from build123d import *

# Parameters (mm, degrees)
REVOLUTION_ANGLE = 100
FILLET_R         = 8
PAD_DEPTH        = 8
POCKET_DEPTH     = 2
CHAMFER_SIZE     = 1
SKETCH005_W      = 3
SKETCH005_H      = 7
POCKET001_DEPTH  = 81.861582
POCKET002_DEPTH  = 78.501
FILLET001_R      = 3
FILLET002_R      = 1


with BuildPart() as part:
    # Sketch → Revolution (revolve, symmetric)
    with BuildSketch(Plane.XY) as revolution_sk:
        with BuildLine():
            ThreePointArc((28, 223.488706), (0, 250), (-28, 223.488706))
            Line((-34.75, 100), (-28, 223.488706))
            Line((-34.75, 100), (-32.5, 100))
            Line((-32.5, 100), (-25.552843, 224))
            ThreePointArc((25.552843, 224), (0, 248.161305), (-25.552843, 224))
            Line((25.552843, 224), (32.5, 100))
            Line((32.5, 100), (34.75, 100))
            Line((34.75, 100), (28, 223.488706))
        make_face()
    revolve(axis=Axis((0, 0, 0), (1, 0, 0)), revolution_arc=REVOLUTION_ANGLE / 2)
    revolve(revolution_sk.sketch, axis=Axis((0, 0, 0), (-1, 0, 0)), revolution_arc=REVOLUTION_ANGLE / 2)

    # Fillet
    fillet_edges = [part.edges().sort_by_distance(p)[0] for p in [
        (33.625, 64.278761, 76.604444),
        (-33.625, 64.278761, 76.604444),
    ]]
    fillet(fillet_edges, radius=FILLET_R)

    # Sketch002 (on Face5 of Fillet) → Pad (new body)
    with BuildSketch(Plane(origin=(0, 0, 0), x_dir=(1, 0, 0), z_dir=(0, -0.766044, 0.642788))):
        Polygon((-43.394171, 132.697505), (-46.5, 121.106395), (-33.248819, 107.855214), (-31, 145.091677), align=None)
        Polygon((43.394171, 132.697505), (46.5, 121.106395), (33.248819, 107.855214), (31, 145.091677), align=None)
        Polygon((28, 194.106395), (32, 198.106395), (32, 206.106395), (28, 210.106395), (24, 206.106395), (24, 198.106395), align=None)
        Polygon((-28, 194.106395), (-24, 198.106395), (-24, 206.106395), (-28, 210.106395), (-32, 206.106395), (-32, 198.106395), align=None)
    extrude(amount=-PAD_DEPTH)

    # Sketch003 (on Face47 of Pad) → Pocket (cut)
    with BuildSketch(Plane(origin=(0, 0, 0), x_dir=(1, 0, 0), z_dir=(0, -0.766044, 0.642788))):
        Polygon((35, 146.869795), (45, 97.88), (47.939388, 98.48), (37.939388, 147.469795), align=None)
        Polygon((-47.939388, 98.48), (-45, 97.88), (-35, 146.869795), (-37.939388, 147.469795), align=None)
    extrude(amount=-POCKET_DEPTH, mode=Mode.SUBTRACT)

    # Chamfer
    chamfer_edges = [part.edges().sort_by_distance(p)[0] for p in [
        (42.094426, 81.707526, 97.375238),
        (38.89944, 82.126736, 97.874832),
        (-38.89944, 82.126736, 97.874832),
        (-42.094426, 81.707526, 97.375238),
    ]]
    chamfer(chamfer_edges, length=CHAMFER_SIZE)

    # Sketch005 (on Face6 of Chamfer) → Pocket001 (cut, through all)
    with BuildSketch(Plane(origin=(0, 6.128356, -5.142301), x_dir=(-1, 0, 0), z_dir=(0, 0.766044, -0.642788))):
        with Locations((-36.047712, 125.078524)):
            Rectangle(SKETCH005_W, SKETCH005_H)
        with Locations((36.047712, 125.078524)):
            Rectangle(SKETCH005_W, SKETCH005_H)
    extrude(amount=-POCKET001_DEPTH, mode=Mode.SUBTRACT)

    # Sketch006 (on Face54 of Pocket001) → Pocket002 (cut, through all)
    with BuildSketch(Plane(origin=(-32, 0, 0), x_dir=(0, -1, 0), z_dir=(-1, 0, 0))):
        Polygon((-140.408225, 149.728159), (-136.657552, 145.044949), (-134.315947, 146.920285), (-138.06662, 151.603495), align=None)
    extrude(amount=-POCKET002_DEPTH, mode=Mode.SUBTRACT)

    # Fillet001
    fillet001_edges = [part.edges().sort_by_distance(p)[0] for p in [
        (46.5, 80.909868, 90.201731),
        (43.394171, 88.36049, 99.081036),
        (-43.394171, 88.36049, 99.081036),
        (-46.5, 80.909868, 90.201731),
    ]]
    fillet(fillet001_edges, radius=FILLET001_R)

    # Fillet002
    fillet002_edges = [part.edges().sort_by_distance(p)[0] for p in [
        (32, 135.546815, 155.315508),
        (32, 130.404514, 149.187153),
        (-32, 130.404514, 149.187153),
        (-32, 135.546815, 155.315508),
    ]]
    fillet(fillet002_edges, radius=FILLET002_R)


solid = part.part
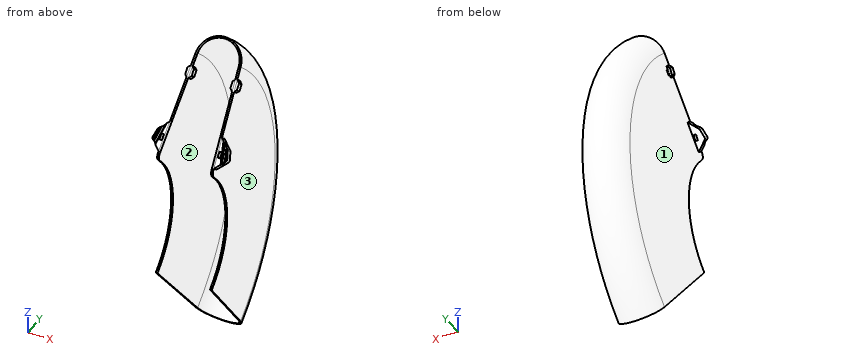
Can you work these out from the model? Positions are in its coordinate system, mm. Face numbers are marked on the shaded views. Give positions to 0.01 mm unless a question says otherwise; leave off trailing zeros. Order: outer loops, then holes, each group sorted by start corner. A loop starts at its lowest first (then second) coordinate and runs counter-clockwise, first axis right, second up. Notation, with made-up numbers: M 69,53 L 120,53 A15 cw 120,79 Z; hole C -3,11.25 d9. An arc over 180 degrees is marked long. Use a Markdown table: item, result. Add a question column.
Item 1: Suppose I cut it at A-A (x = -15). List the corners of the cut face in (y, z) for me.
Item 2: Will these pins go through, and if not, where does the flat tip stop? pin 1 (3.5 mm diameter, centred on y = 133, z = 150, fed in from +X); pin 2 (12.5 mm diameter, centred on y = 135, z = 152.5, fed in from -X); pin 3 (5 mm diameter, centred on y = 171.5, z = -60, fed in from -X).
Item 3: We'd pull the mould along X, two halves only. Please class the marked faces 1, 2 and 3: +X half, -X half, draft (parallel to the pull), parting line (faces both ways), or undercut.
Item 4: If I drill on L1, parallel to X at y = 172, z = 112.5; L2, parallel to X at y = 182, z = -80.5; L3, parallel to Z at x = 10, y = 179, over which ranges is the centre line in solid material (lowest first)? Write a range as [from, to].
Answer sheet:
| question | item | result |
|---|---|---|
| 1 | outline | M 156.39,-186.38 L 157.9,-188.18 A245.65 ccw 157.9,188.18 L 156.39,186.38 A243.3 cw Z |
| 2 | pin 1 | stops at x = 32 |
| 2 | pin 2 | stops at x = -32 |
| 2 | pin 3 | stops at x = -30.42 |
| 3 | face 1 | -X half |
| 3 | face 2 | undercut |
| 3 | face 3 | +X half |
| 4 | L1 | x = [-28.98, -26.59], [26.59, 28.98] |
| 4 | L2 | x = [-29.34, -26.95], [26.95, 29.34] |
| 4 | L3 | z = [-171.87, -168.93], [168.93, 171.87] |
